from build123d import *

# Parameters (mm, degrees)
F0_W     = 40
F0_H     = 40
F1_DEPTH = 10
F2_W     = 20
F2_H     = 29
F3_DEPTH = 5
F4_W     = 15
F4_H     = 5.5
F5_DEPTH = 20
F6_R     = 1.45
F7_DEPTH = 53.2


# Not quite as in the source:
# - a feature names something its author has since deleted; it is built from what else it names


with BuildPart() as f1:
    # F0 (on Top) → F1 (new body)
    with BuildSketch(Plane.XY):
        Rectangle(F0_W, F0_H)
    extrude(amount=F1_DEPTH)

    # F2 (on face) → F3 (join)
    with BuildSketch(Plane(origin=(0, 0, 0), x_dir=(1, 0, 0), z_dir=(0, 0, -1))):
        with Locations((-10, 0)):
            Rectangle(F2_W, F2_H)
    extrude(amount=F3_DEPTH)

    # F4 (on face) → F5 (join)
    with BuildSketch(Plane(origin=(0, 0, 0), x_dir=(1, 0, 0), z_dir=(0, 0, -1))):
        with Locations((12.5, 17.25)):
            Rectangle(F4_W, F4_H)
        with Locations((12.5, -17.25)):
            Rectangle(F4_W, F4_H)
    extrude(amount=F5_DEPTH)

    # F6 (on face) → F7 (cut)
    with BuildSketch(Plane.XZ.offset(20)):
        with Locations((12.5, -15)):
            Circle(F6_R)
    extrude(amount=-F7_DEPTH, mode=Mode.SUBTRACT)


solid = f1.part
Here's how the part is built. I have some questions about the finished solid (model axes, mm). A direction names the side the tool comes from. Give positions to 0.01 mm unless a question says otherwise; leave off trailing zeros. Write each loop counter-clockwise with the first axis right and the second up, starting at its lowest first coordinate (ties: lowest second). Pieces come first, ordered by that corner, then holes. Notation, with made-up numbers: (62.5, 57) -> (75.5, 57) arc R26 ccw to (75.5, 93) -> close; hole circle Ø6 at (-29.75, 50). An arc over 180 degrees is marked (long way). Use one line per item in the form item = value. Start each with the question number.
1. Will these pins go through, and if not, where does the flat tip stop? pin 1 Ø2 at (y, z) = (10, -0.5) entering from +X; pin 2 Ø1.7 at (x, z) = (12.5, -15) entering from +Y; pin 3 Ø4 at (x, z) = (-11.5, -3.5) entering from +Y; pin 4 Ø10 at (x, y) = (-7.5, -10.5) entering from -Z.
2. Imagine slicing it at B-B on y = 15.5. List the corners of the cut face in (x, z) for me, plus the area to 3 significant figures.
3. Imagine slicing it at A-A on x = 12.5. List the corners of the cut face in (y, z) for me.
4. Imagine slicing it at D-D on z = -10.25. List the corners of the cut face in (x, y) for me.
5. Imagine slicing it at C-C on z = -15. List the corners of the cut face in (x, y) for me.
6. If I drill on L1, parallel to Y at x = 14, z = -8.75; L2, parallel to Z at x = -5, y = -1.5; L3, parallel to Z at x = 18.5, y = -11, over which ranges is the centre line in solid material (lowest first)?
7. On a 3-axis mill with a long thin cutter (end or side, diameter ignored), from which of +Z, -Z, +X, -X, +Y, -Y can I reach the whole of each face in a straight line? I mean faces 4 (the face through (12, -14.5, -10)), 5 (the face through (0, 0, -2)), 6 (the face through (-10, 14.5, -2)), 7 (the face through (-10, -14.5, -2)), 8 (the face through (5, -17, -10)). Say none if no direction works.
8. Thinking about a two-plate mould opening in X: for faces 1 (the face through (0, 0, 10)), 2 (the face through (20, 0, 2)), 3 (the face through (11.05, -17.29, -14.94)), which applies, +X half, -X half, draft (parallel to the pull), parting line (faces both ways), or undercut?
Entries:
q1.pin_1 = 20
q1.pin_2 = through
q1.pin_3 = 14.5
q1.pin_4 = -5
q2.outline = (-20, 0) -> (5, 0) -> (5, -20) -> (20, -20) -> (20, 10) -> (-20, 10) -> close; hole circle Ø2.9 at (12.5, -15)
q2.area = 693 mm²
q3.outline = (-20, -20) -> (-14.5, -20) -> (-14.5, -16.45) -> (-20, -16.45) -> close; (-20, -13.55) -> (-14.5, -13.55) -> (-14.5, 0) -> (14.5, 0) -> (14.5, -13.55) -> (20, -13.55) -> (20, 10) -> (-20, 10) -> close; (14.5, -20) -> (20, -20) -> (20, -16.45) -> (14.5, -16.45) -> close
q4.outline = (5, -20) -> (20, -20) -> (20, -14.5) -> (5, -14.5) -> close; (5, 14.5) -> (20, 14.5) -> (20, 20) -> (5, 20) -> close
q5.outline = (5, -20) -> (11.05, -20) -> (11.05, -14.5) -> (5, -14.5) -> close; (5, 14.5) -> (11.05, 14.5) -> (11.05, 20) -> (5, 20) -> close; (13.95, -20) -> (20, -20) -> (20, -14.5) -> (13.95, -14.5) -> close; (13.95, 14.5) -> (20, 14.5) -> (20, 20) -> (13.95, 20) -> close
q6.L1 = -20 to -14.5, 14.5 to 20
q6.L2 = -5 to 10
q6.L3 = 0 to 10
q7.face_4 = -Z, +X
q7.face_5 = -Z, +X, +Y, -Y
q7.face_6 = -Z, -X, +Y
q7.face_7 = -Z, -X, -Y
q7.face_8 = -Z, -X, +Y, -Y
q8.face_1 = draft
q8.face_2 = +X half
q8.face_3 = undercut
